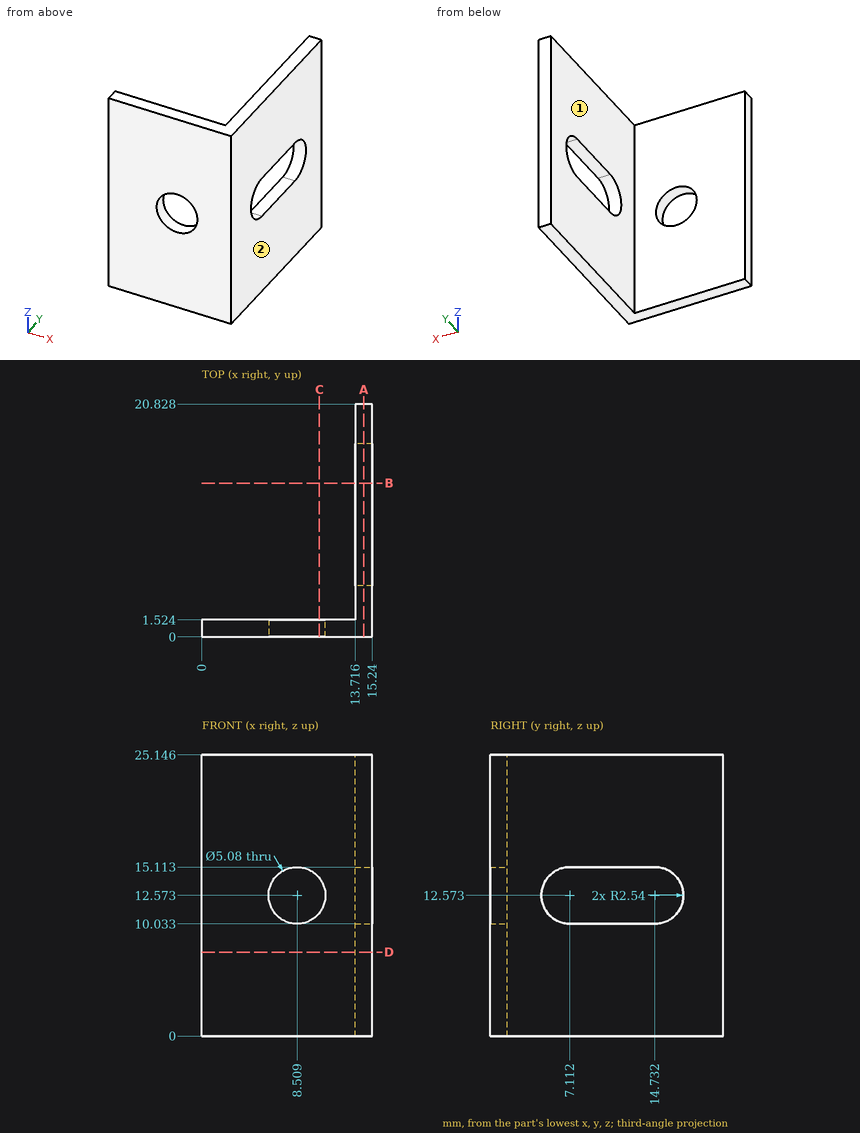
Could you check a few things on this drawing? It's one solid part, dimensions in mm from its lowest x, y, z. A direction names the side the tool comes from. Coordinates: 2 decimals unless noted, no trailing zeros. Order: outer loops, then holes, each group sorted by start corner. A loop starts at its lowest first (then second) coordinate and runs counter-clockwise, first axis right, second up. Notation, with made-up numbers: (5, -16.5) - (22, -16.5) arc R22 cw to (22, 12.5) - close; hole circle Ø4 at (10.25, 38). An arc over 180 degrees is marked (long way). Answer as a JSON object with one key per item and string values. Group by question number.
Q1. Will these pins go through, and if not, where does the flat tip stop? P1, Ø12, axis at y = 8.5, z = 11, coming from the -X side; P2, Ø4, axis at x = 8.509, z = 12.573, coming from the -Y side; P3, Ø3, axis at x = 5, z = 20.5, coming from the +Y side.
Q2. Imagine slicing it at D-D (z = 7.5). Please give me the cut outline in (x, y).
Q3. On a 3-axis mill with a long thin cutter (end or side, diameter ignored), from which of +Z, -Z, +X, -X, +Y, -Y can I reach the whole of each face in a straight line? I mean the marked faces 1 and 2. Say none if no direction works.
Q4. Imagine slicing it at C-C (x = 10.5). Please give me the cut outline in (y, z).
Q5. I need wall thicknesses on line 1 (Y direction, x = 4.5, z = 3); line 2 (X direction, y = 7.5, z = 21.75). Which ranges of each line are inside material? Lowest first, please. Write a range as from..to.
Q6. Imagine slicing it at A-A (x = 14.5). Please give me the cut outline in (y, z), and give its area (3 significant figures).
Q7. Imagine slicing it at B-B (y = 13.75). Please give me the cut outline in (x, z).
Determined:
{
 "1": {"P1": "stops at x = 13.72", "P2": "passes through", "P3": "stops at y = 1.52"},
 "2": {"outline": "(0, 0) - (15.24, 0) - (15.24, 20.83) - (13.72, 20.83) - (13.72, 1.52) - (0, 1.52) - close"},
 "3": {"face 1": "+Z, -Z, -X, +Y", "face 2": "+Z, -Z, +X, +Y, -Y"},
 "4": {"outline": "(0, 0) - (1.52, 0) - (1.52, 11) - (0, 11) - close; (0, 14.15) - (1.52, 14.15) - (1.52, 25.15) - (0, 25.15) - close"},
 "5": {"line 1": "y = 0..1.52", "line 2": "x = 13.72..15.24"},
 "6": {"outline": "(0, 0) - (20.83, 0) - (20.83, 25.15) - (0, 25.15) - close; hole (7.11, 10.03) - (14.73, 10.03) arc R2.54 ccw to (14.73, 15.11) - (7.11, 15.11) arc R2.54 ccw to start", "area": "465 mm2"},
 "7": {"outline": "(13.72, 0) - (15.24, 0) - (15.24, 10.03) - (13.72, 10.03) - close; (13.72, 15.11) - (15.24, 15.11) - (15.24, 25.15) - (13.72, 25.15) - close"}
}
